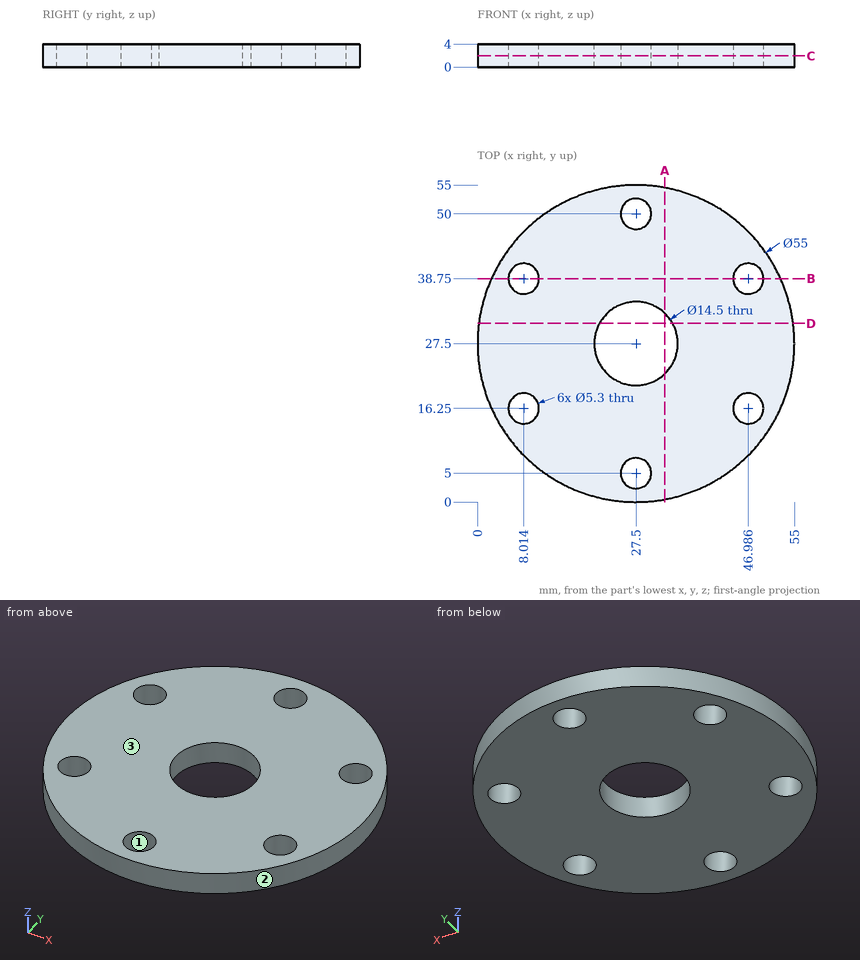
Here's the drawing with two shaded views (mm, measured from the low corner). I have some questions. Round coordinates to 2 decimals unless told otherwise and drop trailing zeros. Loops run counter-clockwise (first coordinate to the right, second up) from the corner with the lowest first, then second, coordinate; pieces in that order, holes last.
1. Will these pins go through, and if not, where does the flat tip stop? pin 1 (2 mm diameter, centred on x = 18.5, z = 2, fed in from +Y); pin 2 (2 mm diameter, centred on y = 10, z = 1, fed in from +X).
Answers:
pin 1: stops at y = 53.81
pin 2: stops at x = 49.5
2. Suppose I cut it at C-C, the plane z = 1.95. Give the number of separate pieces and of enclosed holes in the cut face, and give its area (3 significant figures).
Answers:
separate pieces: 1
enclosed holes: 7
area: 2,080 mm2
3. Suppose I cut it at B-B, the plane y = 38.75. Please give me the cut outline in (x, z) (1 decimal).
Answers:
outline: (2.4, 0) - (5.4, 0) - (5.4, 4) - (2.4, 4) - close; (10.7, 0) - (44.3, 0) - (44.3, 4) - (10.7, 4) - close; (49.6, 0) - (52.6, 0) - (52.6, 4) - (49.6, 4) - close
4. Thinking about a two-plate mould opening in X: for the marked faces 1, 2 and 3, which applies, released by +X, released by -X, zero draft, split by the parting line, or undercut?
Answers:
face 1: undercut
face 2: split by the parting line
face 3: zero draft
5. Suppose I cut it at A-A, the plane x = 32.5. Please give me the cut outline in (y, z).
Answers:
outline: (0.46, 0) - (22.25, 0) - (22.25, 4) - (0.46, 4) - close; (32.75, 0) - (54.54, 0) - (54.54, 4) - (32.75, 4) - close
6. If I drill on probe 1 along Y at (x, z) = (27.5, 1.2); probe 2 along Y at (x, z) = (45.5, 3.05) (1 decimal); probe 3 along X at (y, z) = (17.5, 1.95), over which ranges is the centre line in solid material (lowest first)?
Answers:
probe 1: y = 0 to 2.35, 7.65 to 20.25, 34.75 to 47.35, 52.65 to 55
probe 2: y = 6.7 to 14.1, 18.4 to 36.6, 40.9 to 48.3
probe 3: x = 1.88 to 5.68, 10.35 to 44.65, 49.32 to 53.12
7. Suppose I cut it at D-D, the plane y = 31. Please give me the cut outline in (x, z).
Answers:
outline: (0.22, 0) - (21.15, 0) - (21.15, 4) - (0.22, 4) - close; (33.85, 0) - (54.78, 0) - (54.78, 4) - (33.85, 4) - close
